Autodesk Inventor part; units mm, degrees
ref_plane "YZ Plane" through (0, 0, 0) normal (1, 0, 0) x (0, 1, 0)
ref_plane "XZ Plane" through (0, 0, 0) normal (0, 1, 0) x (-1, 0, 0)
ref_plane "XY Plane" through (0, 0, 0) normal (0, 0, 1) x (1, 0, 0)
sketch "Sketch1" plane through (0, 0, 0) normal (0, 0, 1) x (1, 0, 0)
  arc A0 (11.6951, -1.7956) -> (0, 0) centre (4.624, -8.8667) ccw
  line L0 (11.6951, -1.7956) -> (21.2005, -11.301)
  arc A1 (21.2005, -11.301) -> (22.9683, -12.0332) centre (22.9683, -9.5332) ccw
  line L1 (22.9683, -12.0332) -> (26.5038, -12.0332)
  arc A2 (26.5038, -12.0332) -> (29.0038, -9.5332) centre (26.5038, -9.5332) ccw
  line L2 (29.0038, -9.5332) -> (29.0038, -5.9977)
  arc A3 (29.0038, -5.9977) -> (28.2716, -4.2299) centre (26.5038, -5.9977) ccw
  line L3 (28.2716, -4.2299) -> (18.7662, 5.2754)
  arc A4 (16.9706, 16.9706) -> (18.7662, 5.2754) centre (25.8373, 12.3465) ccw
  arc A5 (16.9706, 16.9706) -> (16.9706, 53.963) centre (-18.4962, 35.4668) ccw
  arc A6 (18.7662, 65.6581) -> (16.9706, 53.963) centre (25.8373, 58.587) ccw
  line L4 (18.7662, 65.6581) -> (28.2716, 75.1635)
  arc A7 (28.2716, 75.1635) -> (29.0038, 76.9312) centre (26.5038, 76.9312) ccw
  line L5 (29.0038, 76.9312) -> (29.0038, 80.4668)
  arc A8 (29.0038, 80.4668) -> (26.5038, 82.9668) centre (26.5038, 80.4668) ccw
  line L6 (26.5038, 82.9668) -> (22.9683, 82.9668)
  arc A9 (22.9683, 82.9668) -> (21.2005, 82.2345) centre (22.9683, 80.4668) ccw
  line L7 (21.2005, 82.2345) -> (11.6951, 72.7291)
  arc A10 (0, 70.9335) -> (11.6951, 72.7291) centre (4.624, 79.8002) ccw
  arc A11 (0, 70.9335) -> (-36.9924, 70.9335) centre (-18.4962, 35.4668) ccw
  arc A12 (-48.6875, 72.7291) -> (-36.9924, 70.9335) centre (-41.6164, 79.8002) ccw
  line L8 (-48.6875, 72.7291) -> (-58.1929, 82.2345)
  arc A13 (-58.1929, 82.2345) -> (-59.9607, 82.9668) centre (-59.9607, 80.4668) ccw
  line L9 (-59.9607, 82.9668) -> (-63.4962, 82.9668)
  arc A14 (-63.4962, 82.9668) -> (-65.9962, 80.4668) centre (-63.4962, 80.4668) ccw
  line L10 (-65.9962, 80.4668) -> (-65.9962, 76.9312)
  arc A15 (-65.9962, 76.9312) -> (-65.264, 75.1635) centre (-63.4962, 76.9312) ccw
  line L11 (-65.264, 75.1635) -> (-55.7586, 65.6581)
  arc A16 (-53.9629, 53.963) -> (-55.7586, 65.6581) centre (-62.8296, 58.587) ccw
  arc A17 (-53.9629, 53.963) -> (-53.963, 16.9706) centre (-18.4962, 35.4668) ccw
  arc A18 (-55.7586, 5.2754) -> (-53.963, 16.9706) centre (-62.8296, 12.3465) ccw
  line L12 (-55.7586, 5.2754) -> (-65.264, -4.2299)
  arc A19 (-65.264, -4.2299) -> (-65.9962, -5.9977) centre (-63.4962, -5.9977) ccw
  line L13 (-65.9962, -5.9977) -> (-65.9962, -9.5332)
  arc A20 (-65.9962, -9.5332) -> (-63.4962, -12.0332) centre (-63.4962, -9.5332) ccw
  line L14 (-63.4962, -12.0332) -> (-59.9607, -12.0332)
  arc A21 (-59.9607, -12.0332) -> (-58.1929, -11.301) centre (-59.9607, -9.5332) ccw
  line L15 (-58.1929, -11.301) -> (-48.6875, -1.7956)
  arc A22 (-36.9924, 0) -> (-48.6875, -1.7956) centre (-41.6164, -8.8667) ccw
  arc A23 (-36.9924, 0) -> (-18.9962, -4.5301) centre (-18.4962, 35.4668) ccw
  arc A24 (-18.9962, -4.5301) -> (-17.9962, -4.5301) centre (-18.4962, -4.5332) ccw
  arc A25 (-17.9962, -4.5301) -> (0, 0) centre (-18.4962, 35.4668) ccw
  circle A26 centre (-49.9962, 3.9668) radius 3
  circle A27 centre (-49.9962, 66.9668) radius 3
  circle A28 centre (13.0038, 3.9668) radius 3
  circle A29 centre (13.0038, 66.9668) radius 3
  circle A30 centre (-18.4962, 35.4668) radius 36
extrude "Extrusion1" add sketch "Sketch1" along normal blind 400
sketch "Sketch2" plane through (0, 0, 400) normal (0, 0, 1) x (1, 0, 0)
  circle A0 centre (-18.4962, 35.4668) radius 36
  circle A1 centre (13.0038, 66.9668) radius 3
  circle A2 centre (13.0038, 3.9668) radius 3
  circle A3 centre (-49.9962, 66.9668) radius 3
  circle A4 centre (-49.9962, 3.9668) radius 3
  arc A5 (-17.9962, -4.5301) -> (0, 0) centre (-18.4962, 35.4668) ccw
  arc A6 (11.6951, -1.7956) -> (0, 0) centre (4.624, -8.8667) ccw
  line L0 (21.2005, -11.301) -> (11.6951, -1.7956)
  arc A7 (21.2005, -11.301) -> (22.9683, -12.0332) centre (22.9683, -9.5332) ccw
  line L1 (26.5038, -12.0332) -> (22.9683, -12.0332)
  arc A8 (26.5038, -12.0332) -> (29.0038, -9.5332) centre (26.5038, -9.5332) ccw
  line L2 (29.0038, -5.9977) -> (29.0038, -9.5332)
  arc A9 (29.0038, -5.9977) -> (28.2716, -4.2299) centre (26.5038, -5.9977) ccw
  line L3 (18.7662, 5.2754) -> (28.2716, -4.2299)
  arc A10 (16.9706, 16.9706) -> (18.7662, 5.2754) centre (25.8373, 12.3465) ccw
  arc A11 (16.9706, 16.9706) -> (16.9706, 53.963) centre (-18.4962, 35.4668) ccw
  arc A12 (18.7662, 65.6581) -> (16.9706, 53.963) centre (25.8373, 58.587) ccw
  line L4 (28.2716, 75.1635) -> (18.7662, 65.6581)
  arc A13 (28.2716, 75.1635) -> (29.0038, 76.9312) centre (26.5038, 76.9312) ccw
  line L5 (29.0038, 80.4668) -> (29.0038, 76.9312)
  arc A14 (29.0038, 80.4668) -> (26.5038, 82.9668) centre (26.5038, 80.4668) ccw
  line L6 (22.9683, 82.9668) -> (26.5038, 82.9668)
  arc A15 (22.9683, 82.9668) -> (21.2005, 82.2345) centre (22.9683, 80.4668) ccw
  line L7 (11.6951, 72.7291) -> (21.2005, 82.2345)
  arc A16 (0, 70.9335) -> (11.6951, 72.7291) centre (4.624, 79.8002) ccw
  arc A17 (0, 70.9335) -> (-36.9924, 70.9335) centre (-18.4962, 35.4668) ccw
  arc A18 (-48.6875, 72.7291) -> (-36.9924, 70.9335) centre (-41.6164, 79.8002) ccw
  line L8 (-58.1929, 82.2345) -> (-48.6875, 72.7291)
  arc A19 (-58.1929, 82.2345) -> (-59.9607, 82.9668) centre (-59.9607, 80.4668) ccw
  line L9 (-63.4962, 82.9668) -> (-59.9607, 82.9668)
  arc A20 (-63.4962, 82.9668) -> (-65.9962, 80.4668) centre (-63.4962, 80.4668) ccw
  line L10 (-65.9962, 76.9312) -> (-65.9962, 80.4668)
  arc A21 (-65.9962, 76.9312) -> (-65.264, 75.1635) centre (-63.4962, 76.9312) ccw
  line L11 (-55.7586, 65.6581) -> (-65.264, 75.1635)
  arc A22 (-53.9629, 53.963) -> (-55.7586, 65.6581) centre (-62.8296, 58.587) ccw
  arc A23 (-53.9629, 53.963) -> (-53.963, 16.9706) centre (-18.4962, 35.4668) ccw
  arc A24 (-55.7586, 5.2754) -> (-53.963, 16.9706) centre (-62.8296, 12.3465) ccw
  line L12 (-65.264, -4.2299) -> (-55.7586, 5.2754)
  arc A25 (-65.264, -4.2299) -> (-65.9962, -5.9977) centre (-63.4962, -5.9977) ccw
  line L13 (-65.9962, -9.5332) -> (-65.9962, -5.9977)
  arc A26 (-65.9962, -9.5332) -> (-63.4962, -12.0332) centre (-63.4962, -9.5332) ccw
  line L14 (-59.9607, -12.0332) -> (-63.4962, -12.0332)
  arc A27 (-59.9607, -12.0332) -> (-58.1929, -11.301) centre (-59.9607, -9.5332) ccw
  line L15 (-48.6875, -1.7956) -> (-58.1929, -11.301)
  arc A28 (-36.9924, 0) -> (-48.6875, -1.7956) centre (-41.6164, -8.8667) ccw
  arc A29 (-36.9924, 0) -> (-18.9962, -4.5301) centre (-18.4962, 35.4668) ccw
  arc A30 (-18.9962, -4.5301) -> (-17.9962, -4.5301) centre (-18.4962, -4.5332) ccw
extrude "Extrusion2" cut sketch "Sketch2" against normal blind 250
properties part number "X95_150mm"
Here's how the part is built. I have some questions about the finished solid (model axes, mm). A direction names the side the tool comes from. Round coordinates to 2 decimals unless told otherwise and drop trailing zeros. Write each loop counter-clockwise with the first axis right and the second up, starting at its lowest first coordinate (ties: lowest second). Pieces come first, ordered by that corner, then holes.
1. I need wall thicknesses on L1, parallel to Y at x = 11, z = 35.5; L2, parallel to Y at x = -48.5, z = 72.5; L3, parallel to Y at x = 5, z = 143. Which ranges of each line are inside material? Lowest first, please.
2. Suppose I cut it at B-B (x = -27.5). List the corners of the cut face in (y, z) for me.
3. Will these pins go through, and if not, where does the flat tip stop? pin 1 Ø2 at (y, z) = (8, 92.5) entering from -X; pin 2 Ø1.5 at (y, z) = (67, 49) entering from -X; pin 3 Ø2 at (y, z) = (50.5, 113) entering from -X.
4. Suppose I cut it at C-C (z = 21.5). State how many separate pieces and enclosed holes the cut face has, and give its area (3 significant figures).
5. For faces 4 (the flat face through (23.45, 70.34, 73.95)), 5 (the flat face through (-60.445, 0.589, 73.95)), 6 (the flat face through (-53.374, 77.415, 73.95)), 7 (the flat face through (16.4, -6.5, 74)), which set-ups out of +Z, -Z, +X, -X, +Y, -Y let a thin tool reach every point of the face, with its end or its side?
6. If we mould it in two halves opening along Y, with no side actions, what happens to faces 1 (the cylindrical face through (-43.222, 1.004, 73.95)), 2 (the flat face through (23.585, 0.456, 73.95)), 3 (the flat face through (-54, 43, 150))? For each: released by +Y, released by -Y, zero draft, split by the parting line, or undercut.
7. Suppose I cut it at A-A (y = 26). List the corners of the cut face in (x, z) for me, and give its area (3 significant figures).
Answer sheet:
1. L1: y = -1.16 to 1.73, 6.2 to 14.83, 56.11 to 64.73, 69.2 to 72.1
1. L2: y = -1.61 to 1.37, 6.57 to 15.57, 55.36 to 64.37, 69.57 to 72.55
1. L3: y = 1.13 to 8.19, 62.74 to 69.81
2. outline: (-3.51, 0) - (0.61, 0) - (0.61, 150) - (-3.51, 150) - close; (70.32, 0) - (74.44, 0) - (74.44, 150) - (70.32, 150) - close
3. pin 1: stops at x = -54.38
3. pin 2: stops at x = -57.85
3. pin 3: stops at x = -55.95
4. separate pieces: 1
4. enclosed holes: 5
4. area: 1,920 mm2
5. face 4: +Z, -Z, +X
5. face 5: +Z, -Z, -X
5. face 6: +Z, -Z, +Y
5. face 7: +Z, -Z, -Y
6. face 1: released by -Y
6. face 2: undercut
6. face 3: zero draft
7. outline: (-57.36, 0) - (-53.23, 0) - (-53.23, 150) - (-57.36, 150) - close; (16.24, 0) - (20.37, 0) - (20.37, 150) - (16.24, 150) - close
7. area: 1,240 mm2
